Geometry: final body of the model. Coordinates: model frame, mm. A direction names the side the tool comes from. Round coordinates to 2 decimals unless told otherwise and drop trailing zeros. Loops run counter-clockwise (first coordinate to the right, second up) from the corner with the lowest first, then second, coordinate; pieces in that order, holes last. Notation, with made-up numbers: (-12.75, 83) -> (-3.75, 83) arc R21 ccw to (-3.75, 95) -> close; hole circle Ø8 at (59.25, 31). An arc over 180 degrees is marked (long way). Answer in a Markdown table with one row per item.
```python
from build123d import *

# Parameters (mm, degrees)
F0_W     = 203.2
F0_H     = 203.2
F1_DEPTH = 406.4
F2_W     = 177.8
F2_H     = 177.8
F3_DEPTH = 63.5
F4_R     = 9.525
F5_DEPTH = 205.74
F6_W     = 50.8
F6_H     = 63.5
F7_DEPTH = 228.6
F8_W     = 73.0317101263
F8_H     = 190.5
F9_DEPTH = 101.6
F10_R    = 5.08


with BuildPart() as f1:
    # F0 (on Top) → F1 (new body)
    with BuildSketch(Plane.XY):
        Rectangle(F0_W, F0_H)
    extrude(amount=F1_DEPTH)

    # F2 (on face) → F3 (cut)
    with BuildSketch(Plane.XY.offset(406.4)):
        Rectangle(F2_W, F2_H)
    extrude(amount=-F3_DEPTH, mode=Mode.SUBTRACT)

    # F4 (on face) → F5 (cut)
    with BuildSketch(Plane.XZ.offset(101.6)):
        with Locations((-69.85, 374.65)):
            Circle(F4_R)
        with Locations((69.85, 374.65)):
            Circle(F4_R)
    extrude(amount=-F5_DEPTH, mode=Mode.SUBTRACT)

    # F6 (on face) → F7 (cut)
    with BuildSketch(Plane.YZ.offset(101.6)):
        with Locations((0, 374.65)):
            Rectangle(F6_W, F6_H)
    extrude(amount=-F7_DEPTH, mode=Mode.SUBTRACT)

    # F8 (on face) → F9 (join)
    with BuildSketch(Plane.XY):
        Rectangle(F8_W, F8_H)
    extrude(amount=-F9_DEPTH)

    # F10
    f10_edges = [f1.edges().sort_by_distance(p)[0] for p in [
        (-101.6, 101.6, 203.2),
        (-101.6, -101.6, 203.2),
        (101.6, 101.6, 203.2),
        (101.6, 63.5, 406.4),
        (0, 101.6, 406.4),
        (-101.6, 63.5, 406.4),
        (-101.6, -63.5, 406.4),
        (0, -101.6, 406.4),
        (101.6, -101.6, 203.2),
        (101.6, 0, 0),
        (0, -101.6, 0),
        (0, 101.6, 0),
        (-101.6, 0, 0),
        (-88.9, -88.9, 374.65),
        (-88.9, 88.9, 374.65),
        (88.9, -88.9, 374.65),
        (88.9, 88.9, 374.65),
        (36.515855, 0, -101.6),
        (-36.515855, 0, -101.6),
    ]]
    fillet(f10_edges, radius=F10_R)


solid = f1.part
```
Item 1: Set-up query: faces 4 (the flat face through (95, 25.4, 374)), 5 (the flat face through (-36.516, -1, -48)), 6 (the flat face through (-1, -95.25, -50)), 7 (the flat face through (-1, -88.9, 375)). Return all of +Z, -Z, +X, -X, +Y, -Y with unobstructed straight access to the full face (end or side cutting, diameter ignored); none if empty.
Ans:
| item | result |
|---|---|
| face 4 | +Z, +X, -X |
| face 5 | -Z, -X, +Y, -Y |
| face 6 | -Z, +X, -X, -Y |
| face 7 | +Z |
Item 2: Section query B-B, the plane y = 55.5. Output: boundary loops of the cut face in (x, z).
Ans:
| item | result |
|---|---|
| outline | (-101.6, 5.08) arc R5.08 ccw to (-96.52, 0) -> (-36.52, 0) -> (-36.52, -96.52) arc R5.08 ccw to (-31.44, -101.6) -> (31.44, -101.6) arc R5.08 ccw to (36.52, -96.52) -> (36.52, 0) -> (96.52, 0) arc R5.08 ccw to (101.6, 5.08) -> (101.6, 401.32) arc R5.08 ccw to (96.52, 406.4) -> (88.9, 406.4) -> (88.9, 342.9) -> (-88.9, 342.9) -> (-88.9, 406.4) -> (-96.52, 406.4) arc R5.08 ccw to (-101.6, 401.32) -> close |
Item 3: Section query D-D, the plane y = -12. Output: boundary loops of the cut face in (x, z).
Ans:
| item | result |
|---|---|
| outline | (-101.6, 5.08) arc R5.08 ccw to (-96.52, 0) -> (-36.52, 0) -> (-36.52, -96.52) arc R5.08 ccw to (-31.44, -101.6) -> (31.44, -101.6) arc R5.08 ccw to (36.52, -96.52) -> (36.52, 0) -> (96.52, 0) arc R5.08 ccw to (101.6, 5.08) -> (101.6, 342.9) -> (-101.6, 342.9) -> close |
Item 4: First-contact query: P1, Ø12, axis at x = -80, y = -77.5, coming from the +Z side; P2, Ø1.5, axis at y = 67, z = -34, coming from the +X side; P3, Ø12, axis at y = -32, z = -15.5, coming from the -X side. Flat tips, straight axial feed; report the tip coordinate or a pass-through.
Ans:
| item | result |
|---|---|
| P1 | z = 342.9 |
| P2 | x = 36.52 |
| P3 | x = -36.52 |
Item 5: Section query A-A, the plane x = 69.85. Output: boundary loops of the cut face in (y, z) (3 decimals).
Ans:
| item | result |
|---|---|
| outline | (-101.6, 5.08) arc R5.08 ccw to (-96.52, 0) -> (96.52, 0) arc R5.08 ccw to (101.6, 5.08) -> (101.6, 365.125) -> (88.9, 365.125) -> (88.9, 342.9) -> (-88.9, 342.9) -> (-88.9, 365.125) -> (-101.6, 365.125) -> close; (-101.6, 384.175) -> (-88.9, 384.175) -> (-88.9, 406.4) -> (-96.52, 406.4) arc R5.08 ccw to (-101.6, 401.32) -> close; (88.9, 384.175) -> (101.6, 384.175) -> (101.6, 401.32) arc R5.08 ccw to (96.52, 406.4) -> (88.9, 406.4) -> close |
Item 6: Mould query, pull axis Y, two halves, no side actions, for faces 1 (the cylindrical face through (68.61, -95.339, 384.094)), 2 (the flat face through (-1, 95.25, -50)), 3 (the flat face through (88.9, -55, 375)). Classes: released by +Y, released by -Y, zero draft, split by the parting line, or undercut.
Ans:
| item | result |
|---|---|
| face 1 | zero draft |
| face 2 | released by +Y |
| face 3 | undercut |
Item 7: Ray query, L1, parallel to X at y = 92, z = 374; L2, parallel to Z at x = 69.85, y = 96.5 (3 decimals); L3, parallel to Z at x = 69, y = 93. Return the intervals inside material, ascending.
Ans:
| item | result |
|---|---|
| L1 | -101.6 to -79.35, -60.35 to 60.35, 79.35 to 101.6 |
| L2 | 0 to 365.125, 384.175 to 406.4 |
| L3 | 0 to 365.16, 384.14 to 406.4 |
Item 8: Section query C-C, the plane z = 374.65. State how many separate pieces and enclosed holes the cut face has, and give its area (3 significant figures).
Ans:
| item | result |
|---|---|
| separate pieces | 6 |
| enclosed holes | 0 |
| area | 7,420 mm2 |
